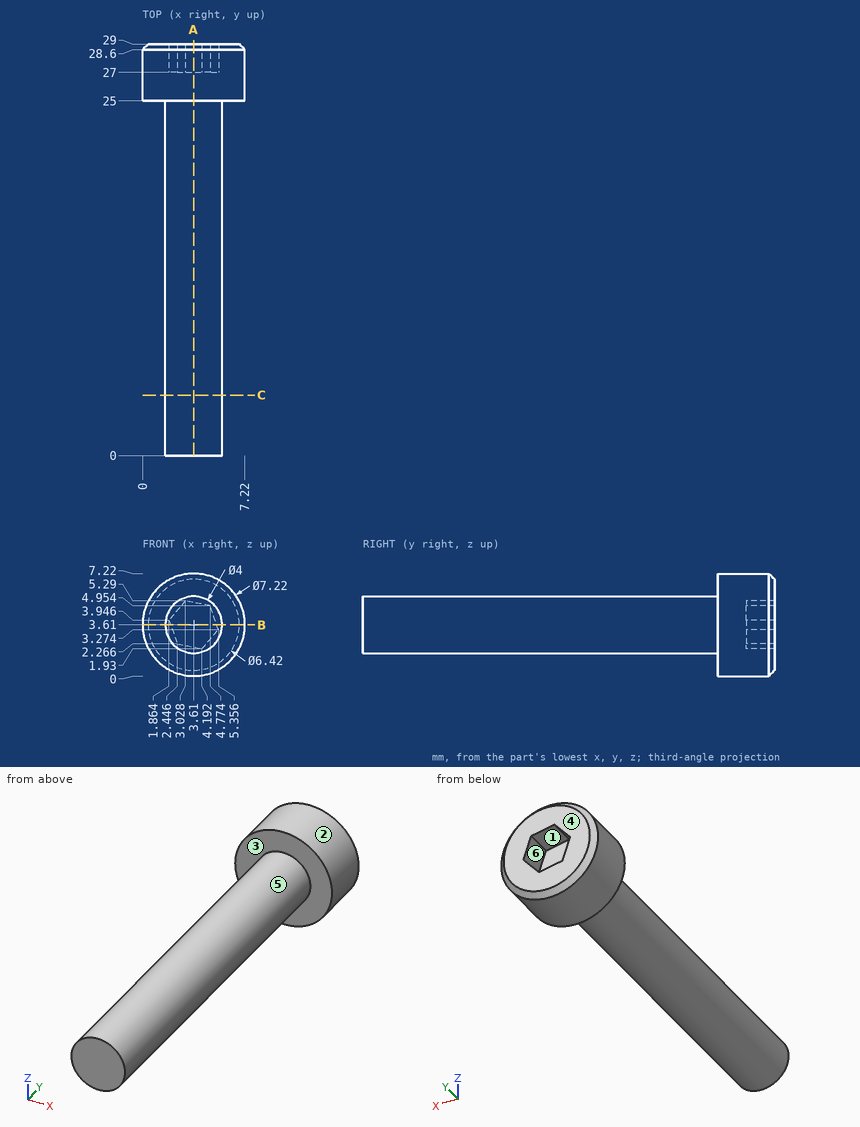
Study the drawing (mm; zero at the part's minimum x, y, z) and answer. A direction names the side the tool comes from. Give positions to 0.01 mm unless a question says otherwise; leave off trailing zeros. Order: outer loops, then holes, each group sorted by start corner. A loop starts at its lowest first (then second) coordinate and runs counter-clockwise, first axis right, second up.
1) Find section A-A on x = 3.61. Write down the section's boundary in (y, z), then the cut area to 3 significant figures.
Reported:
outline: (0, 1.61) - (25, 1.61) - (25, 0) - (28.6, 0) - (29, 0.4) - (29, 2.04) - (27, 2.04) - (27, 5.18) - (29, 5.18) - (29, 6.82) - (28.6, 7.22) - (25, 7.22) - (25, 5.61) - (0, 5.61) - close
area: 122 mm2
2) Find section B-B on z = 3.61. Write down the section's boundary in (x, y), then the cut area to 3 significant figures.
Reported:
outline: (0, 25) - (1.61, 25) - (1.61, 0) - (5.61, 0) - (5.61, 25) - (7.22, 25) - (7.22, 28.6) - (6.82, 29) - (5.24, 29) - (5.24, 27) - (1.98, 27) - (1.98, 29) - (0.4, 29) - (0, 28.6) - close
area: 122 mm2
3) Determine the mould class of the marked faces 4, 5 and 6 for opening direction Z: pulls with the +Z half, pulls with the -Z half, needs draft (parallel to the pull), parting line crosses it, or undercut.
Reported:
face 4: needs draft
face 5: parting line crosses it
face 6: undercut
4) For the marked faces 1, 2 and 3, determine the directions among +Z, -Z, +X, -X, +Y, -Y from which every point of the face is accessible in a straight line to the end or side of a thin tool.
Reported:
face 1: +Y
face 2: +Y, -Y
face 3: -Y
5) Given P1, Ø2, axis at x = 4.5, y = 23, coming from the +Z side; P2, Ø1, axis at x = 3, z = 3.5, coming from the +Y side; P3, Ø1.5, axis at y = 16, z = 6.5, coming from the -X side; P4, Ø2, axis at x = 1.5, y = 25.5, coming from the +Z side (1 decimal), each flat-ended and moving along its own axis, determine where each tip first touches the part or whether it passes through.
Reported:
P1: stops at z = 5.61
P2: stops at y = 27
P3: passes through
P4: stops at z = 7
6) Find section C-C on y = 4.25. Write down the section's boundary in (x, z), then the cut area to 3 significant figures.
Reported:
outline: circle Ø4 at (3.61, 3.61)
area: 12.6 mm2
7) Consider line 1 along X through (y, z) = (17.5, 3.5); line 2 along Y through (x, z) = (1.75, 4.75); line 3 along Z through (x, y) = (3.75, 6.5) (1 decimal). Determine where each line is inside the solid, lowest interval first.
Reported:
line 1: x = 1.61 to 5.61
line 2: y = 25 to 29
line 3: z = 1.6 to 5.6
